Input: part model. Units: mm. Frame: model coordinates. Give positions to 0.01 mm unless a question says otherwise; leave off trailing zeros. Write each loop counter-clockwise with the first axis right and the second up, starting at its lowest first coordinate (ties: lowest second). Pieces come first, ordered by that corner, then holes.
```python
from build123d import *

# Parameters (mm, degrees)
BOSS_EXTRUDE1_DEPTH       = 123.825
SKETCH11_W                = 1.5875
SKETCH11_H                = 4.7625
CUT_EXTRUDE2_DEPTH        = 10.525
F_6_32_TAPPED_HOLE1_D     = 2.7051
F_6_32_TAPPED_HOLE1_DEPTH = 9.398


with BuildPart() as part:
    # Sketch1 → Boss-Extrude1 (new body, symmetric)
    with BuildSketch(Plane.XY):
        Polygon((0, 4.7625), (0, -4.7625), (9.525, -4.7625), (9.525, -3.175), (1.5875, -3.175), (1.5875, 3.175), (9.525, 3.175), (9.525, 4.7625), align=None)
    extrude(amount=BOSS_EXTRUDE1_DEPTH, both=True)

    # Sketch11 → Cut-Extrude2 (cut, through all)
    with BuildSketch(Plane.ZY):
        with Locations((-120.49125, 0)):
            Rectangle(SKETCH11_W, SKETCH11_H)
        with Locations((-114.14125, 0)):
            Rectangle(SKETCH11_W, SKETCH11_H)
    extrude(amount=-CUT_EXTRUDE2_DEPTH, mode=Mode.SUBTRACT)

    # #6-32 Tapped Hole1
    with Locations(Plane.ZY):
        with Locations((-100.6475, 0), (-87.80859375, 0), (-74.9696875, 0), (-62.13078125, 0), (-49.291875, 0), (-36.45296875, 0), (-23.6140625, 0), (-10.77515625, 0), (2.06375, 0), (14.90265625, 0), (27.7415625, 0), (40.58046875, 0), (53.419375, 0), (66.25828125, 0), (79.0971875, 0), (91.93609375, 0)):
            Hole(F_6_32_TAPPED_HOLE1_D / 2, depth=F_6_32_TAPPED_HOLE1_DEPTH)


solid = part.part
```
Q1. Mould query, pull axis Y, two halves, no side actions, for faces 1 (the flat face through (5, 4.762, 2)), 2 (the flat face through (6, -3.175, 2)), 3 (the flat face through (0, -2, 2)), 4 (the flat face through (5, -4.762, 2)). Classes: +Y half, -Y half, draft (parallel to the pull), parting line (faces both ways), or undercut.
Q2. Pin query (flat end, axial travel): pin 1 (4.5 mm diameter, centred on y = 0, z = -36.45, fed in from -X); pin 2 (3 mm diameter, centred on y = 1, z = -66.5, fed in from +X). Return the tip coordinate at first contact, or that it passes through.
Q3. Material intervals for line 1 along Z through (x, y) = (1.25, -2.25) (1 decimal); line 2 along Y through (x, z) = (3.75, 22) (1 decimal); line 3 along X through (y, z) = (-0.5, 12), sorted ascending.
Q4. Section A-A, the plane x = 3.25. Return the cut outline in (y, z) (1 decimal).
Solutions:
1. face 1: +Y half
1. face 2: undercut
1. face 3: draft
1. face 4: -Y half
2. pin 1: stops at x = 0
2. pin 2: stops at x = 1.59
3. line 1: z = -123.8 to -121.3, -119.7 to -114.9, -113.3 to 123.8
3. line 2: y = -4.8 to -3.2, 3.2 to 4.8
3. line 3: x = 0 to 1.59
4. outline: (-4.8, -123.8) - (-3.2, -123.8) - (-3.2, 123.8) - (-4.8, 123.8) - close; (3.2, -123.8) - (4.8, -123.8) - (4.8, 123.8) - (3.2, 123.8) - close
